from build123d import *

# Parameters (mm, degrees)
SKETCH1_W           = 50
SKETCH1_H           = 86.65
BOSS_EXTRUDE1_DEPTH = 7.5
SKETCH7_W           = 5.5
SKETCH7_H           = 62.4
CUT_EXTRUDE5_DEPTH  = 5.95
SKETCH11_R          = 2.1
CUT_EXTRUDE8_DEPTH  = 8.5
SKETCH12_R          = 2.1
CUT_EXTRUDE10_DEPTH = 8.5
SKETCH13_W          = 86.65
SKETCH13_H          = 7.5
BOSS_EXTRUDE2_DEPTH = 1
SKETCH14_W          = 86.65
SKETCH14_H          = 7.5
CUT_EXTRUDE11_DEPTH = 10


with BuildPart() as part:
    # Sketch1 → Boss-Extrude1 (new body)
    with BuildSketch(Plane(origin=(0, 0, 0), x_dir=(1, 0, 0), z_dir=(0, 1, 0))):
        Rectangle(SKETCH1_W, SKETCH1_H)
    extrude(amount=BOSS_EXTRUDE1_DEPTH)

    # Sketch7 → Cut-Extrude5 (cut)
    with BuildSketch(Plane(origin=(0, 7.5, 0), x_dir=(1, 0, 0), z_dir=(0, 1, 0))):
        with Locations((-8.15, -3.875)):
            Rectangle(SKETCH7_W, SKETCH7_H)
    extrude(amount=-CUT_EXTRUDE5_DEPTH, mode=Mode.SUBTRACT)

    # Sketch11 → Cut-Extrude8 (cut, through all)
    with BuildSketch(Plane(origin=(0, 7.5, 0), x_dir=(1, 0, 0), z_dir=(0, 1, 0))):
        with Locations((17.982, 35.325)):
            Circle(SKETCH11_R)
        with Locations((-10.018, 35.325)):
            Circle(SKETCH11_R)
    extrude(amount=-CUT_EXTRUDE8_DEPTH, mode=Mode.SUBTRACT)

    # Sketch12 → Cut-Extrude10 (cut, through all)
    with BuildSketch(Plane(origin=(0, 7.5, 0), x_dir=(1, 0, 0), z_dir=(0, 1, 0))):
        with Locations((20.25, 10.821)):
            Circle(SKETCH12_R)
        with Locations((20.25, -38.229)):
            Circle(SKETCH12_R)
    extrude(amount=-CUT_EXTRUDE10_DEPTH, mode=Mode.SUBTRACT)

    # Sketch13 → Boss-Extrude2 (add)
    with BuildSketch(Plane(origin=(25, 0, 0), x_dir=(0, 0, -1), z_dir=(1, 0, 0))):
        with Locations((0, 3.75)):
            Rectangle(SKETCH13_W, SKETCH13_H)
    extrude(amount=BOSS_EXTRUDE2_DEPTH)

    # Sketch14 → Cut-Extrude11 (cut)
    with BuildSketch(Plane.ZY.offset(25)):
        with Locations((0, 3.75)):
            Rectangle(SKETCH14_W, SKETCH14_H)
    extrude(amount=-CUT_EXTRUDE11_DEPTH, mode=Mode.SUBTRACT)


solid = part.part
Here's how the part is built. I have some questions about the finished solid (model axes, mm). A direction names the side the tool comes from. Give positions to 0.01 mm unless a question says otherwise; leave off trailing zeros. Write each loop counter-clockwise with the first axis right and the second up, starting at its lowest first coordinate (ties: lowest second). Pieces come first, ordered by that corner, then holes. Notation, with made-up numbers: (37.25, -27) -> (52.25, -27) arc R19 cw to (52.25, -14) -> close; hole circle Ø4 at (49.25, -29). An arc over 180 degrees is marked (long way). Use one line per item in the form item = value. Start each with the question number.
1. Will this pin go through, and if not, where does the flat tip stop? pin 1 Ø2.5 at (x, z) = (20.25, 38.229) entering from +Y.
2. If I drill on L1, parallel to Z at x = 20.25, y = 5.25 (3 decimals); L2, parallel to X at y = 4.5, z = -24; L3, parallel to Z at x = -9, y = 5 (3 decimals), over which ranges is the centre line in solid material (lowest first)?
3. On a 3-axis mill with a long thin cutter (end or side, diameter ignored), from which of +Z, -Z, +X, -X, +Y, -Y can I reach the whole of each face in a straight line? I mean faces 1 (the face through (-5.4, 5, 4)), 2 (the face through (-15, 4, -1)). Say none if no direction works.
4. Thinking about a two-plate mould opening in Z: for faces 3 (the face through (5, 4, -43.325)), 4 (the face through (16.316, 3.802, -34.047)), 5 (the face through (26, 4, 1)), which applies, +Z half, -Z half, draft (parallel to the pull), parting line (faces both ways), or undercut?
5. Imagine slicing it at C-C on y = 6.5. List the corners of the cut face in (x, z) for me (3 decimals).
6. Imagine slicing it at A-A on x = -7. List the corners of the cut face in (y, z) for me (3 decimals).
7. Imagine slicing it at B-B on z = 17.5. List the corners of the cut face in (x, y) for me, plus the area to 3 significant figures.
Entries:
q1.pin_1 = through
q2.L1 = -43.325 to -12.921, -8.721 to 36.129, 40.329 to 43.325
q2.L2 = -15 to -10.9, -5.4 to 26
q2.L3 = -43.325 to -37.162, -33.488 to -27.325, 35.075 to 43.325
q3.face_1 = +Y
q3.face_2 = +Z, -Z, -X, +Y, -Y
q4.face_3 = -Z half
q4.face_4 = undercut
q4.face_5 = draft
q5.outline = (-15, -43.325) -> (26, -43.325) -> (26, 43.325) -> (-15, 43.325) -> close; hole circle Ø4.2 at (-10.018, -35.325); hole (-10.9, -27.325) -> (-5.4, -27.325) -> (-5.4, 35.075) -> (-10.9, 35.075) -> close; hole circle Ø4.2 at (17.982, -35.325); hole circle Ø4.2 at (20.25, -10.821); hole circle Ø4.2 at (20.25, 38.229)
q6.outline = (0, -43.325) -> (7.5, -43.325) -> (7.5, -27.325) -> (1.55, -27.325) -> (1.55, 35.075) -> (7.5, 35.075) -> (7.5, 43.325) -> (0, 43.325) -> close
q7.outline = (-15, 0) -> (26, 0) -> (26, 7.5) -> (-5.4, 7.5) -> (-5.4, 1.55) -> (-10.9, 1.55) -> (-10.9, 7.5) -> (-15, 7.5) -> close
q7.area = 275 mm²
